The model under review builds one solid part; all positions refer to its coordinate system, in mm. A direction names the side the tool comes from. Coordinates: 2 decimals unless noted, no trailing zeros. Write each loop counter-clockwise with the first axis right and the second up, starting at its lowest first coordinate (ties: lowest second). Pieces come first, ordered by that corner, then holes. Notation, with made-up numbers: M 68,-35 L 123,-35 A26 ccw 123,-3 Z; hole C -17,86 d4. An arc over 180 degrees is marked long. Answer as CSV lines item,"result". Start each with the question number.
from build123d import *

# Parameters (mm, degrees)
BOX001_W                    = 10
BOX001_H                    = 10
BOX001_DEPTH                = 18
PAD001_DEPTH                = 1
BOX_W                       = 1
BOX_H                       = 4
BOX_DEPTH                   = 62
BOX_PLACEMENT_ANGLE         = 340
CYLINDER_R                  = 2
CYLINDER_DEPTH              = 67
CYLINDER_PLACEMENT_ANGLE    = 340
CYLINDER001_R               = 4
CYLINDER001_DEPTH           = 60
CYLINDER001_PLACEMENT_ANGLE = 20
SKETCH_R                    = 2.527902
PAD_DEPTH                   = 10
FILLET_R                    = 2
FILLET001_R                 = 2
FILLET002_R                 = 2
FILLET004_R                 = 1


with BuildPart() as box001:
    # Box001 → Box001 (new body)
    with BuildSketch(Plane(origin=(-4.48, -1.55, 0), x_dir=(0, -1, 0), z_dir=(0, 0, 1))):
        with Locations((5, 5)):
            Rectangle(BOX001_W, BOX001_H)
    extrude(amount=BOX001_DEPTH)


with BuildPart() as body001:
    # Sketch001 → Pad001 (new body, symmetric)
    with BuildSketch(Plane.YZ):
        Polygon((11.126045, 25.12734), (5.15667, 9.780665), (10.086619, 0), (14.214679, 32.616486), align=None)
    extrude(amount=PAD001_DEPTH, both=True)


with BuildPart() as box:
    # Box → Box (new body)
    with BuildSketch(Plane.XY):
        with Locations((0.5, 2)):
            Rectangle(BOX_W, BOX_H)
    extrude(amount=BOX_DEPTH)


with BuildPart() as box_1:
    # Box placement: moved
    add(box.part.moved(Location((0, -5.296136, 2.991813))).rotate(Axis((0, -5.296136, 2.991813), (1, 0, 0)), BOX_PLACEMENT_ANGLE))


with BuildPart() as cylinder:
    # Cylinder → Cylinder (new body)
    with BuildSketch(Plane.XY):
        Circle(CYLINDER_R)
    extrude(amount=CYLINDER_DEPTH)


with BuildPart() as cylinder_1:
    # Cylinder placement: moved
    add(cylinder.part.moved(Location((0, -2.318081, -1.61877))).rotate(Axis((0, -2.318081, -1.61877), (1, 0, 0)), CYLINDER_PLACEMENT_ANGLE))


with BuildPart() as cylinder001:
    # Cylinder001 → Cylinder001 (new body)
    with BuildSketch(Plane.XY):
        Circle(CYLINDER001_R)
    extrude(amount=CYLINDER001_DEPTH)


with BuildPart() as cylinder001_1:
    # Cylinder001 placement: moved
    add(cylinder001.part.moved(Location((0, -0.95, 2.14))).rotate(Axis((0, -0.95, 2.14), (-1, 0, 0)), CYLINDER001_PLACEMENT_ANGLE))


with BuildPart() as cut002:
    # Sketch → Pad (new body)
    with BuildSketch(Plane.XY):
        with BuildLine():
            ThreePointArc((-11.024148, 4.03498), (-16.038919, -1.856194), (-8.310522, -1.501592))
            Line((-8.310522, -1.501592), (0, -1.501592))
            Line((8.310522, -1.501592), (0, -1.501592))
            ThreePointArc((8.310522, -1.501592), (16.038919, -1.856194), (11.024148, 4.03498))
            Line((11.024148, 4.03498), (3.534046, 10.276075))
            Line((3.534046, 10.276075), (0, 10.276075))
            Line((-3.534046, 10.276075), (0, 10.276075))
            Line((-11.024148, 4.03498), (-3.534046, 10.276075))
        make_face()
        with Locations((-12.251753, 0)):
            Circle(SKETCH_R, mode=Mode.SUBTRACT)
        with Locations((12.251753, 0)):
            Circle(SKETCH_R, mode=Mode.SUBTRACT)
    extrude(amount=PAD_DEPTH)

    # Fusion: union Cylinder001
    add(cylinder001_1.part)

    # Cut: cut Cylinder
    add(cylinder_1.part, mode=Mode.SUBTRACT)

    # Cut001: cut Box
    add(box_1.part, mode=Mode.SUBTRACT)

    # Fillet
    fillet_edges = [cut002.edges().sort_by_distance(p)[0] for p in [
        (-1.866147, 5.675875, 10),
    ]]
    fillet(fillet_edges, radius=FILLET_R)

    # Fusion001: union Body001
    add(body001.part)

    # Fillet001
    fillet001_edges = [cut002.edges().sort_by_distance(p)[0] for p in [
        (-3.534046, 10.276075, 5),
    ]]
    fillet(fillet001_edges, radius=FILLET001_R)

    # Fillet002
    fillet002_edges = [cut002.edges().sort_by_distance(p)[0] for p in [
        (3.534046, 10.276075, 5),
    ]]
    fillet(fillet002_edges, radius=FILLET002_R)

    # Fillet004
    fillet004_edges = [cut002.edges().sort_by_distance(p)[0] for p in [
        (1.905002, 10.276075, 10),
        (-1.905002, 10.276075, 10),
    ]]
    fillet(fillet004_edges, radius=FILLET004_R)

    # Cut002: cut Box001
    add(box001.part, mode=Mode.SUBTRACT)


solid = cut002.part
1) Take a section at A-A on x = 14. Give the boundary of the cut face in (y, z).
2) To check wall thickness, follow line 1 (X direction, y = -2.25, z = 9); line 2 (Z direction, x = -8, y = 6); line 3 (Z direction, x = 7, y = 2.75). State the ranges of each line that lie inside material, in increasing order. Write a range as [from, to].
3) Clearance check with flat-ended pins moving along their axes: pin 1 Ø11 at (x, y) = (-10.5, 5) entering from +Z; pin 2 Ø3 at (x, y) = (12.25, 0) entering from +Z; pin 3 Ø3 at (x, z) = (-2.5, 6.5) entering from -Y; pin 4 Ø12 at (y, z) = (19, 34.5) entering from +X. State where each tip first meets the part, or that it passes through.
4) Mouldability with a two-part tool opening along Y and no side actions: class faces 4 (the cylindrical face through (-0.44, 10.62, 28.22)), 5 (the cylindrical face through (-14.777, 0.111, 4.93)), 6 (the flat face through (1, 11, 17)), 7 (the flat face through (-7.61, 6.88, 4.44)) as +Y half, -Y half, draft (parallel to the pull), parting line (faces both ways), or undercut.
5) Tool access review of faces 1 (the cylindrical face through (-3.48, 10.16, 4.56)), 2 (the flat face through (-2, -1.55, 7)), 3 (the flat face through (0, 7, 33)): name each direction out of +Z, -Z, +X, -X, +Y, -Y from which nothing blocks a thin tool from reaching the whole face with its end or side.
6) Take a section at B-B on y = 0. Give the number of separate pieces and of enclosed holes in the cut face, and give its area (3 significant figures).
Results:
1,outline,"M -3.84,0 L -1.83,0 L -1.83,10 L -3.84,10 Z; M 1.83,0 L 3.84,0 L 3.84,10 L 1.83,10 Z"
2,line 1,"x = [-15.82, -13.4], [-11.1, -8.68], [8.68, 11.1], [13.4, 15.82]"
2,line 2,"z = [0, 9.82]"
2,line 3,"z = [0, 10]"
3,pin 1,"stops at z = 10.14"
3,pin 2,"passes through"
3,pin 3,"stops at y = -1.55"
3,pin 4,"stops at x = 3.63"
4,face 4,"undercut"
4,face 5,"undercut"
4,face 6,"draft"
4,face 7,"+Y half"
5,face 1,"-Z, -X, +Y"
5,face 2,"+Z, -Z, -Y"
5,face 3,"+Z, -Y"
6,separate pieces,"4"
6,enclosed holes,"0"
6,area,"221 mm²"
